Verification items for the finished model (mm, model axes). A direction names the side the tool comes from. Round coordinates to 2 decimals unless told otherwise and drop trailing zeros. Write each loop counter-clockwise with the first axis right and the second up, starting at its lowest first coordinate (ties: lowest second). Pieces come first, ordered by that corner, then holes. Notation, with made-up numbers: M 30,15 L 81,15 A27 cw 81,37 Z; hole C -31,-8 d10. An arc over 180 degrees is marked long. One line per question, with ' | ' between items.
Autodesk Inventor part; units mm, degrees
ref_plane "Work Plane1" through (0, 20, 0) normal (0, 1, 0) x (1, 0, 0)
ref_plane "YZ Plane" through (0, 0, 0) normal (1, 0, 0) x (0, 1, 0)
ref_plane "XZ Plane" through (0, 0, 0) normal (0, 1, 0) x (-1, 0, 0)
sketch "Sketch1" plane through (0, 0, 0) normal (0, 1, 0) x (-1, 0, 0)
  line L0 (-21, 21) -> (21, 21)
  line L1 (21, 21) -> (21, -21)
  line L2 (21, -21) -> (-21, -21)
  line L3 (-21, -21) -> (-21, 21)
  line L4 (-21, 21) -> (21, -21) construction
  line L5 (21, 21) -> (-21, -21) construction
  point P0 (0, 0)
  dimension "d0" = 42
  dimension "d1" = 42
extrude "Extrusion1" add sketch "Sketch1" along normal blind 40
ref_plane "Work Plane1" through (0, 20, 0) normal (0, 1, 0) x (1, 0, 0)
sketch "Sketch2" plane through (0, 40, 0) normal (0, 1, 0) x (1, 0, 0)
  line L0 (0, -38.0423) -> (-38.0423, 0)
  line L1 (-38.0423, 0) -> (0, 38.0423)
  line L2 (0, 38.0423) -> (38.0423, 0)
  line L3 (38.0423, 0) -> (0, -38.0423)
  line L4 (0, -38.0423) -> (0, 38.0423) construction
  line L5 (-38.0423, 0) -> (38.0423, 0) construction
  line L6 (-21, 21) -> (-21, -21)
  circle A0 centre (0, 0) radius 250
  dimension "d4" = 53.8
  dimension "d5" = 53.8
  dimension "d6" = 500
extrude "Extrusion2" cut sketch "Sketch2" against normal blind 10
sketch "Sketch3" plane through (0, 20, 0) normal (0, 1, 0) x (1, 0, 0)
  line L0 (-20.9, -20.9) -> (20.9, -20.9)
  line L1 (20.9, -20.9) -> (20.9, 20.9)
  line L2 (20.9, 20.9) -> (-20.9, 20.9)
  line L3 (-20.9, 20.9) -> (-20.9, -20.9)
  line L4 (-21, -21) -> (-21, -17.0423)
  line L5 (21, -21) -> (17.0423, -21)
  line L6 (21, 21) -> (21, 17.0423)
  line L7 (-21, 21) -> (-17.0423, 21)
  circle A0 centre (0, 0) radius 200
  dimension "d9" = 0.1
  dimension "d10" = 0.1
  dimension "d11" = 0.1
  dimension "d12" = 0.1
  dimension "d13" = 400
extrude "Extrusion3" cut sketch "Sketch3" along normal up to surface (10 mm away)
chamfer "Chamfer1" distance 6 angle 45 4 edges at (20.9, 25, 20.9) (20.9, 25, -20.9) (-20.9, 25, 20.9) (-20.9, 25, -20.9)
mirror "Mirror1" about plane through (0, 20, 0) normal (0, 1, 0) of "Extrusion3", "Extrusion2", "Chamfer1"
sketch "Sketch4" plane through (0, 40, 0) normal (0, 1, 0) x (1, 0, 0)
  circle A0 centre (0, 0) radius 11
  dimension "d19" = 22
extrude "Extrusion4" add sketch "Sketch4" along normal blind 2
sketch "Sketch5" plane through (0, 40, 0) normal (0, 1, 0) x (1, 0, 0)
  circle A0 centre (0, 0) radius 11
  line L0 (17.0423, -21) -> (21, -17.0423)
  line L1 (21, -17.0423) -> (21, 17.0423)
  line L2 (21, 17.0423) -> (17.0423, 21)
  line L3 (17.0423, 21) -> (-17.0423, 21)
  line L4 (-17.0423, 21) -> (-21, 17.0423)
  line L5 (-21, 17.0423) -> (-21, -17.0423)
  line L6 (-21, -17.0423) -> (-17.0423, -21)
  line L7 (-17.0423, -21) -> (17.0423, -21)
  circle A1 centre (0, 0) radius 16
  dimension "d22" = 32
extrude "Extrusion5" cut sketch "Sketch5" against normal blind 0.5 contours A1
sketch "Sketch6" plane through (0, 42, 0) normal (0, 1, 0) x (1, 0, 0)
  circle A0 centre (0, 0) radius 3
  dimension "d25" = 6
extrude "Extrusion6" cut sketch "Sketch6" against normal blind 2
sketch "Sketch8" plane through (0, 40, 0) normal (0, 1, 0) x (1, 0, 0)
  circle A0 centre (0, 0) radius 16 construction
  line L0 (17.0423, -21) -> (21, -17.0423) construction
  line L1 (21, -17.0423) -> (21, 17.0423) construction
  line L2 (21, 17.0423) -> (17.0423, 21) construction
  line L3 (17.0423, 21) -> (-17.0423, 21) construction
  line L4 (-17.0423, 21) -> (-21, 17.0423) construction
  line L5 (-21, 17.0423) -> (-21, -17.0423) construction
  line L6 (-21, -17.0423) -> (-17.0423, -21) construction
  line L7 (-17.0423, -21) -> (17.0423, -21) construction
  line L8 (-15.5, -15.5) -> (15.5, -15.5) construction
  line L9 (15.5, -15.5) -> (15.5, 15.5) construction
  line L10 (15.5, 15.5) -> (-15.5, 15.5) construction
  line L11 (-15.5, 15.5) -> (-15.5, -15.5) construction
  line L12 (-15.5, -15.5) -> (15.5, 15.5) construction
  line L13 (15.5, -15.5) -> (-15.5, 15.5) construction
  circle A1 centre (-15.5, 15.5) radius 1.5
  circle A2 centre (15.5, 15.5) radius 1.5
  circle A3 centre (15.5, -15.5) radius 1.5
  circle A4 centre (-15.5, -15.5) radius 1.5
  dimension "d36" = 31
  dimension "d37" = 31
  dimension "d38" = 3
  dimension "d39" = 3
  dimension "d40" = 3
  dimension "d41" = 3
extrude "Extrusion8" cut sketch "Sketch8" against normal blind 5
thread "Thread2"
sketch "Sketch9" plane through (0, 40, 0) normal (0, 1, 0) x (1, 0, 0)
  circle A0 centre (0, 0) radius 2.5
  dimension "d49" = 5
extrude "Extrusion9" add sketch "Sketch9" along normal blind 20
pattern_circular "Circular Pattern2" count 4 over 360 about axis through (0, 40, 0) along (0, 1, 0) of "Extrusion8"
sketch "Sketch10" plane through (0, 60, 0) normal (0, 1, 0) x (1, 0, 0)
  circle A0 centre (0, 0) radius 2.5
  circle A1 centre (0, 0) radius 2.5
  line L0 (-1.5, -2) -> (1.5, -2)
  line L1 (1.5, -2) -> (1.5, -2.5)
  line L2 (1.5, -2.5) -> (-1.5, -2.5)
  line L3 (-1.5, -2.5) -> (-1.5, -2)
  circle A2 centre (0, 0) radius 2.5
  dimension "d55" = 0.5
extrude "Extrusion10" cut sketch "Sketch10" against normal blind 15 contours L0 A0 | A0 L2 L3 | L1 L2 A0 picked at (0.3466, -2.0912)
equation "\"d9\" = d10"
equation "\"d11\" = d10"
equation "\"d12\" = d10"
properties part number "nema17_40mm"
1. Section check B-B, the plane y = 28. Record the cut outline in (x, z).
Results:
outline: M -20.9,-14.9 L -14.9,-20.9 L 14.9,-20.9 L 20.9,-14.9 L 20.9,14.9 L 14.9,20.9 L -14.9,20.9 L -20.9,14.9 Z
2. Go/stop test with flat-tipped pins: P1, Ø10, axis at x = 7, y = 22, coming from the +Z side; P2, Ø5, axis at x = -14, z = -16, coming from the +Y side; P3, Ø1.5, axis at x = 15.5, z = -15.5, coming from the +Y side. Record where each tip stops, or that it passes through.
Results:
P1: stops at z = 20.9 | P2: stops at y = 40 | P3: stops at y = 35
3. Section check D-D, the plane y = 8.5. Record the cut outline in (x, z), then the cut area to 3 significant figures.
Results:
outline: M -21,-17.04 L -17.04,-21 L 17.04,-21 L 21,-17.04 L 21,17.04 L 17.04,21 L -17.04,21 L -21,17.04 Z | area: 1,730 mm2
4. Thickness scan on line 1 (Z direction, x = 0, y = 41.5); line 2 (Z direction, x = 15.5, y = 37.9). Record the ranges inside material, lowest first.
Results:
line 1: z = -11 to -3, -2.5 to 2.5, 3 to 11 | line 2: z = -21 to -17, -14 to 14, 17 to 21
5. Mould release check, pull along Z, two halves, no side actions. Record for faces 1 (the face through (-17, 37.53, -15.57)), 2 (the face through (0, 35, -21)), 3 (the face through (2.3, 42, 2.3)), 4 (the face through (14, 37.53, 15.43)): pulls with the +Z half, pulls with the -Z half, needs draft (parallel to the pull), parting line crosses it, or undercut.
Results:
face 1: undercut | face 2: pulls with the -Z half | face 3: needs draft | face 4: undercut
6. Section check C-C, the plane z = 0. Record the cut outline in (x, y).
Results:
outline: M -21,0 L 21,0 L 21,10 L 20.9,10 L 20.9,30 L 21,30 L 21,40 L 16,40 L 16,39.5 L 11,39.5 L 11,42 L 3,42 L 3,40 L 2.5,40 L 2.5,60 L -2.5,60 L -2.5,40 L -3,40 L -3,42 L -11,42 L -11,39.5 L -16,39.5 L -16,40 L -21,40 L -21,30 L -20.9,30 L -20.9,10 L -21,10 Z
7. Tool access check on faces 5 (the face through (-18.8, 30, -18.8)), 6 (the face through (-17.9, 20.1, 17.9)), 7 (the face through (-16, 35, -16)), 8 (the face through (-20.9, 20, 0)). Record the directions out of +Z, -Z, +X, -X, +Y, -Y that give a thin tool (end or side, any length) a straight path to the whole face; none if there is none.
Results:
face 5: none | face 6: +Z, -X | face 7: +Y | face 8: +Z, -Z, -X
